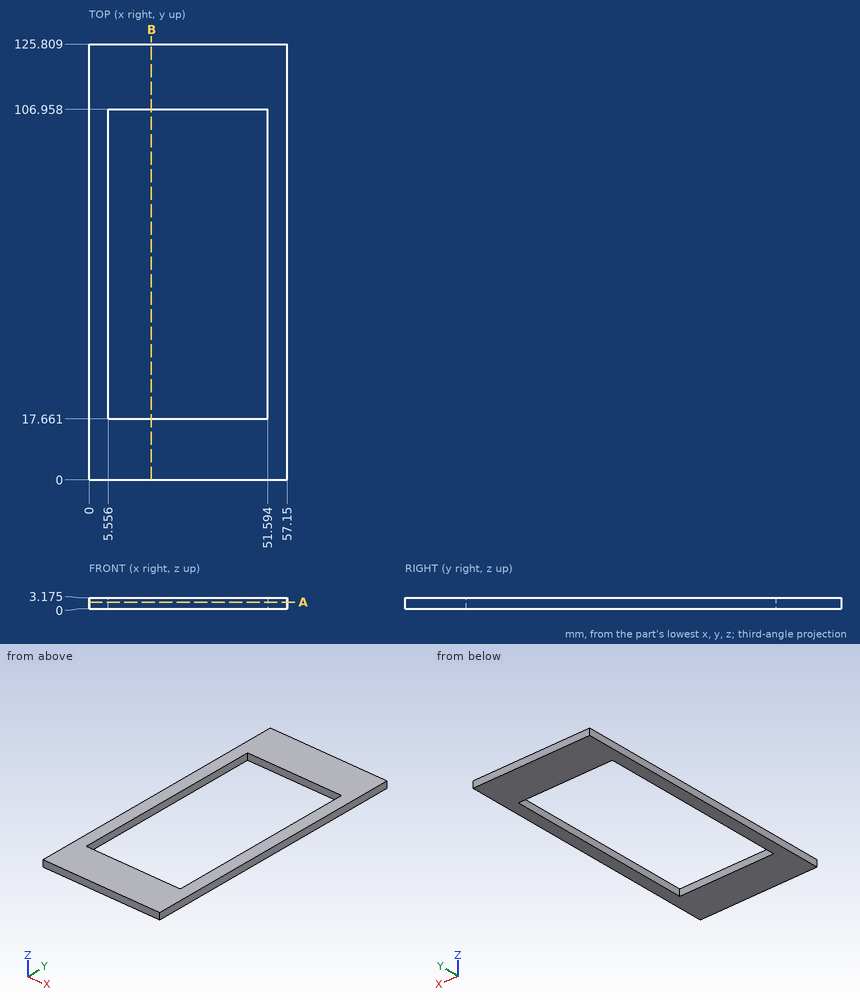
Geometry: see drawing. Coordinates: mm, zero at the bounding-box minimum. Coordinates: 2 decimals unless noted, no trailing zeros. Write each loop counter-clockwise with the first axis right and the second up, starting at its lowest first coordinate (ties: lowest second). Pieces come first, ordered by that corner, then holes.
1) Material intervals for line 1 along X through (y, z) = (60, 1.6); line 2 along Y through (x, z) = (13, 1.65), sorted ascending.
2) Section A-A on z = 2. Output: boundary loops of the cut face in (x, y), and give its area (3 significant figures).
3) Section B-B on x = 18. Output: boundary loops of the cut face in (y, z) (1 decimal).
Check result:
1. line 1: x = 0 to 5.56, 51.59 to 57.15
1. line 2: y = 0 to 17.66, 106.96 to 125.81
2. outline: (0, 0) - (57.15, 0) - (57.15, 125.81) - (0, 125.81) - close; hole (5.56, 17.66) - (51.59, 17.66) - (51.59, 106.96) - (5.56, 106.96) - close
2. area: 3,080 mm2
3. outline: (0, 0) - (17.7, 0) - (17.7, 3.2) - (0, 3.2) - close; (107, 0) - (125.8, 0) - (125.8, 3.2) - (107, 3.2) - close
